Geometry: final body of the model. Coordinates: model frame, mm. Face numbers are marked on the shaded views. Give positions to 0.01 mm unless a question says otherwise; leave off trailing zeros. Write each loop counter-clockwise with the first axis right and the second up, starting at its lowest first coordinate (ties: lowest second). Pieces come first, ordered by that corner, then holes.
Q1. Cut plane C-C on y = 5.5. Return the cut outline in (x, z), plus the area to 3 significant figures.
Q2. Line query: L1, parallel to Z at x = 10, y = 7.25; L2, parallel to Z at x = 68, y = 14.5; L3, parallel to Y at x = 56.5, z = 12. Output: solid intervals per line, ascending.
Q3. Pin query (flat end, axial travel): pin 1 (1 mm diameter, centred on y = 2, z = 2.5, fed in from -X); pin 2 (1 mm diameter, centred on x = 84.5, z = -10.5, fed in from +Y); pin 3 (4 mm diameter, centred on x = 20.5, y = 4, fed in from -Z). Return the tip coordinate at first contact, or that it passes through.
Q4. Cut plane D-D on z = -5.25. Return the cut outline in (x, y), plus the area to 3 significant figures.
Q5. Draft query along Z for the marked faces 1 and 2. Return one class per face: pulls with the +Z half, pulls with the -Z half, needs draft (parallel to the pull), parting line crosses it, or undercut.
Q6. Cut plane B-B on x = 22. Return the cut outline in (y, z).
Q7. Cut plane A-A on y = 10.75. Return the cut outline in (x, z).
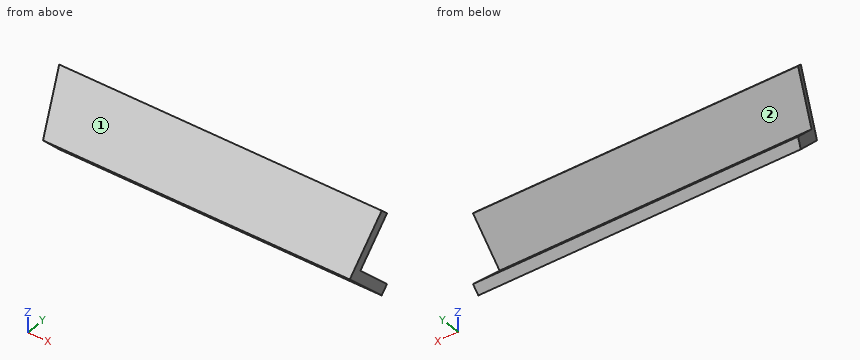
```python
from build123d import *

# Parameters (mm, degrees)
BOSS_EXTRUDE1_DEPTH = 101.6
SKETCH2_W           = 26.940768364
SKETCH2_H           = 16.724030672
CUT_EXTRUDE1_DEPTH  = 99.46706905


with BuildPart() as part:
    # Sketch1 → Boss-Extrude1 (new body)
    with BuildSketch(Plane(origin=(0, 0, 0), x_dir=(0, 0, -1), z_dir=(1, 0, 0))):
        Polygon((0, 0), (-13.470384182, 13.470384182), (-11.225320151, 15.715448212), (0, 4.490128061), (11.225320151, 15.715448212), (13.470384182, 13.470384182), align=None)
    extrude(amount=BOSS_EXTRUDE1_DEPTH)

    # Sketch2 → Cut-Extrude1 (cut, through all)
    with BuildSketch(Plane(origin=(5.050847696, 1.838358219, 0), x_dir=(0, 0, -1), z_dir=(-0.9396926207859081, -0.34202014332566943, 0))):
        with Locations((0, -6.405675381)):
            Rectangle(SKETCH2_W, SKETCH2_H)
    extrude(amount=CUT_EXTRUDE1_DEPTH, mode=Mode.SUBTRACT)


solid = part.part
```
Data:
1. outline: (3.72, -5.5) - (101.6, -5.5) - (101.6, -1.01) - (3.72, -1.01) - close; (3.72, 1.01) - (101.6, 1.01) - (101.6, 5.5) - (3.72, 5.5) - close
1. area: 879 mm2
2. L1: z = -7.25 to -2.76, 2.76 to 7.25
2. L2: z = -12.44 to -10.01, 10.01 to 12.44
2. L3: y = 12 to 14.94
3. pin 1: stops at x = 4.81
3. pin 2: stops at y = 15.49
3. pin 3: stops at z = -6
4. outline: (2.17, 9.74) - (3.81, 5.25) - (101.6, 5.25) - (101.6, 9.74) - close
4. area: 443 mm2
5. face 1: pulls with the +Z half
5. face 2: undercut
6. outline: (0, 0) - (13.47, -13.47) - (15.72, -11.23) - (4.49, 0) - (15.72, 11.23) - (13.47, 13.47) - close
7. outline: (1.81, -10.75) - (101.6, -10.75) - (101.6, -6.26) - (1.81, -6.26) - close; (1.81, 6.26) - (101.6, 6.26) - (101.6, 10.75) - (1.81, 10.75) - close
